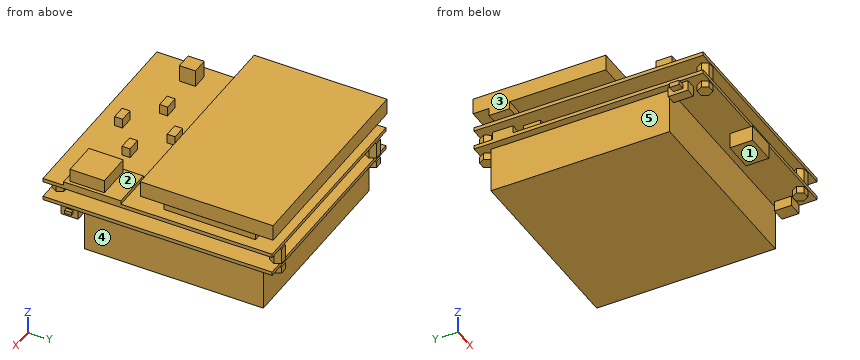
from build123d import *

# Parameters (mm, degrees)
SKETCH001_W   = 91
SKETCH001_H   = 100
PAD_DEPTH     = 1.6
SKETCH002_W   = 84.4
SKETCH002_H   = 78
PAD001_DEPTH  = 20
SKETCH003_W   = 13
SKETCH003_H   = 10
PAD002_DEPTH  = 6.8
SKETCH004_W   = 4.3
SKETCH004_H   = 8.6
PAD003_DEPTH  = 4.6
SKETCH005_W   = 6
SKETCH005_H   = 7.4
PAD004_DEPTH  = 4.4
SKETCH006_W   = 4.2
SKETCH006_H   = 2
PAD005_DEPTH  = 3
SKETCH007_W   = 3
SKETCH007_H   = 1.5
PAD006_DEPTH  = 1.4
PAD007_DEPTH  = 7
SKETCH009_W   = 7
SKETCH009_H   = 9
PAD008_DEPTH  = 3.4
SKETCH010_W   = 5
SKETCH010_H   = 7.4
PAD009_DEPTH  = 2.6
SKETCH011_W   = 91
SKETCH011_H   = 100
PAD010_DEPTH  = 1.6
SKETCH012_W   = 40
SKETCH012_H   = 4
SKETCH012_W_2 = 4
SKETCH012_H_2 = 40
PAD011_DEPTH  = 7.8
SKETCH013_W   = 91
SKETCH013_H   = 58
PAD012_DEPTH  = 7
SKETCH014_W   = 7
SKETCH014_H   = 9
PAD013_DEPTH  = 3.4
PAD014_DEPTH  = 3
SKETCH035_W   = 6
SKETCH035_H   = 3.5
PAD021_DEPTH  = 4.2
SKETCH036_W   = 7
SKETCH036_H   = 7
PAD022_DEPTH  = 7.4
SKETCH037_W   = 18
SKETCH037_H   = 25
PAD023_DEPTH  = 1.6
SKETCH038_W   = 15
SKETCH038_H   = 15
PAD024_DEPTH  = 5.8


with BuildPart() as part:
    # Sketch001 → Pad (new body)
    with BuildSketch(Plane.XY):
        Rectangle(SKETCH001_W, SKETCH001_H)
    extrude(amount=PAD_DEPTH)

    # Sketch002 (on Face5 of Pad) → Pad001 (join)
    with BuildSketch(Plane(origin=(0, 0, 0), x_dir=(1, 0, 0), z_dir=(0, 0, -1))):
        with Locations((0, -5.4)):
            Rectangle(SKETCH002_W, SKETCH002_H)
    extrude(amount=PAD001_DEPTH)

    # Sketch003 (on Face4 of Pad001) → Pad002 (join)
    with BuildSketch(Plane(origin=(0, 0, 0), x_dir=(1, 0, 0), z_dir=(0, 0, -1))):
        with Locations((-0.5, 45.6)):
            Rectangle(SKETCH003_W, SKETCH003_H)
    extrude(amount=PAD002_DEPTH)

    # Sketch004 (on Face4 of Pad002) → Pad003 (join)
    with BuildSketch(Plane(origin=(0, 0, 0), x_dir=(1, 0, 0), z_dir=(0, 0, -1))):
        with Locations((-41.95, 38.3)):
            Rectangle(SKETCH004_W, SKETCH004_H)
    extrude(amount=PAD003_DEPTH)

    # Sketch005 (on Face4 of Pad003) → Pad004 (join)
    with BuildSketch(Plane(origin=(0, 0, 0), x_dir=(1, 0, 0), z_dir=(0, 0, -1))):
        with Locations((41.9, 38.7)):
            Rectangle(SKETCH005_W, SKETCH005_H)
    extrude(amount=PAD004_DEPTH)

    # Sketch006 (on Face14 of Pad004) → Pad005 (join)
    with BuildSketch(Plane(origin=(-44.1, 0, 0), x_dir=(0, -1, 0), z_dir=(-1, 0, 0))):
        with Locations((38.3, -2)):
            Rectangle(SKETCH006_W, SKETCH006_H)
    extrude(amount=PAD005_DEPTH)

    # Sketch007 (on Face12 of Pad005) → Pad006 (join)
    with BuildSketch(Plane.YZ.offset(44.9)):
        with Locations((-38.7, -1.75)):
            Rectangle(SKETCH007_W, SKETCH007_H)
    extrude(amount=PAD006_DEPTH)

    # Sketch008 (on Face5 of Pad006) → Pad007 (join)
    with BuildSketch(Plane.XY.offset(1.6)):
        Polygon((-40, 45.401924), (-37, 45.401924), (-35.5, 48), (-37, 50.598076), (-40, 50.598076), (-41.5, 48), align=None)
        Polygon((39, 45.401924), (40.5, 48), (39, 50.598076), (36, 50.598076), (34.5, 48), (36, 45.401924), align=None)
        Polygon((-37, -49.598076), (-35.5, -47), (-37, -44.401924), (-40, -44.401924), (-41.5, -47), (-40, -49.598076), align=None)
        Polygon((39, -49.598076), (40.5, -47), (39, -44.401924), (36, -44.401924), (34.5, -47), (36, -49.598076), align=None)
    extrude(amount=PAD007_DEPTH)

    # Sketch009 (on Face5 of Pad007) → Pad008 (join)
    with BuildSketch(Plane.XY.offset(1.6)):
        with Locations((-42, 37.5)):
            Rectangle(SKETCH009_W, SKETCH009_H)
    extrude(amount=PAD008_DEPTH)

    # Sketch010 (on Face5 of Pad008) → Pad009 (join)
    with BuildSketch(Plane.XY.offset(1.6)):
        with Locations((-42, 25.3)):
            Rectangle(SKETCH010_W, SKETCH010_H)
    extrude(amount=PAD009_DEPTH)

    # Sketch011 (on Face74 of Pad009) → Pad010 (join)
    with BuildSketch(Plane.XY.offset(8.6)):
        Rectangle(SKETCH011_W, SKETCH011_H)
    extrude(amount=PAD010_DEPTH)

    # Sketch012 (on Face81 of Pad010) → Pad011 (join)
    with BuildSketch(Plane.XY.offset(10.2)):
        with Locations((0, 44)):
            Rectangle(SKETCH012_W, SKETCH012_H)
        with Locations((38.5, 20)):
            Rectangle(SKETCH012_W_2, SKETCH012_H_2)
    extrude(amount=PAD011_DEPTH)

    # Sketch013 (on Face91 of Pad011) → Pad012 (join)
    with BuildSketch(Plane.XY.offset(18)):
        with Locations((1, 22)):
            Rectangle(SKETCH013_W, SKETCH013_H)
    extrude(amount=PAD012_DEPTH)

    # Sketch014 (on Face4 of Pad012) → Pad013 (join)
    with BuildSketch(Plane(origin=(0, 0, 18), x_dir=(1, 0, 0), z_dir=(0, 0, -1))):
        with Locations((-41, -39.5)):
            Rectangle(SKETCH014_W, SKETCH014_H)
    extrude(amount=PAD013_DEPTH)

    # Sketch015 (on Face66 of Pad013) → Pad014 (join)
    with BuildSketch(Plane(origin=(0, 0, 0), x_dir=(1, 0, 0), z_dir=(0, 0, -1))):
        Polygon((-35.5, 47), (-37, 49.598076), (-40, 49.598076), (-41.5, 47), (-40, 44.401924), (-37, 44.401924), align=None)
        Polygon((39, 44.401924), (40.5, 47), (39, 49.598076), (36, 49.598076), (34.5, 47), (36, 44.401924), align=None)
        Polygon((-37, -50.598076), (-35.5, -48), (-37, -45.401924), (-40, -45.401924), (-41.5, -48), (-40, -50.598076), align=None)
        Polygon((39, -50.598076), (40.5, -48), (39, -45.401924), (36, -45.401924), (34.5, -48), (36, -50.598076), align=None)
    extrude(amount=PAD014_DEPTH)

    # Sketch035 (on Face20 of Pad014) → Pad021 (join)
    with BuildSketch(Plane.XY.offset(10.2)):
        with Locations((-15, -28.75)):
            Rectangle(SKETCH035_W, SKETCH035_H)
        with Locations((0, -17.25)):
            Rectangle(SKETCH035_W, SKETCH035_H)
        with Locations((15, -28.75)):
            Rectangle(SKETCH035_W, SKETCH035_H)
        with Locations((0, -40.25)):
            Rectangle(SKETCH035_W, SKETCH035_H)
    extrude(amount=PAD021_DEPTH)

    # Sketch036 (on Face20 of Pad021) → Pad022 (join)
    with BuildSketch(Plane.XY.offset(10.2)):
        with Locations((-37, -30.1)):
            Rectangle(SKETCH036_W, SKETCH036_H)
    extrude(amount=PAD022_DEPTH)

    # Sketch037 (on Face20 of Pad022) → Pad023 (join)
    with BuildSketch(Plane.XY.offset(10.2)):
        with Locations((36.5, -28.5)):
            Rectangle(SKETCH037_W, SKETCH037_H)
    extrude(amount=PAD023_DEPTH)

    # Sketch038 (on Face50 of Pad023) → Pad024 (join)
    with BuildSketch(Plane.XY.offset(11.8)):
        with Locations((36.5, -31.5)):
            Rectangle(SKETCH038_W, SKETCH038_H)
    extrude(amount=PAD024_DEPTH)


solid = part.part
Can you work these out from the model? Positions are in its coordinate system, mm. Face numbers are marked on the shaded views. A direction names the side the tool comes from. Round coordinates to 2 decimals unless told otherwise and drop trailing zeros. Order: outer loops, then holes, each group sorted by start corner. A loop starts at its lowest first (then second) coordinate and runs counter-clockwise, first axis right, second up. Notation, with made-up numbers: (18, 60.25) - (23, 60.25) arc R17 ccw to (23, 70.25) - close; hole circle Ø9 at (15.25, 19). An arc over 180 degrees is marked (long way). Answer in a Markdown table with one row per item.
(1) Suppose I cut it at B-B, the plane x = 22. Please give me the cut outline in (y, z).
From the geometry:
| item | result |
|---|---|
| outline | (-50, 0) - (-33.6, 0) - (-33.6, -20) - (44.4, -20) - (44.4, 0) - (50, 0) - (50, 1.6) - (-50, 1.6) - close; (-50, 8.6) - (50, 8.6) - (50, 10.2) - (-50, 10.2) - close; (-7, 18) - (51, 18) - (51, 25) - (-7, 25) - close |
(2) Suppose I cut it at C-C, the plane y = 8. Please give me the cut outline in (x, z).
From the geometry:
| item | result |
|---|---|
| outline | (-45.5, 0) - (-42.2, 0) - (-42.2, -20) - (42.2, -20) - (42.2, 0) - (45.5, 0) - (45.5, 1.6) - (-45.5, 1.6) - close; (-45.5, 8.6) - (45.5, 8.6) - (45.5, 10.2) - (40.5, 10.2) - (40.5, 18) - (46.5, 18) - (46.5, 25) - (-44.5, 25) - (-44.5, 18) - (36.5, 18) - (36.5, 10.2) - (-45.5, 10.2) - close |
(3) For P1, Ø3, axis at y = 25.5, z = 3, coming from the +X side; P2, Ø4, axis at y = 37.5, z = 11, coming from the -X side; P3, Ø0.8, axis at x = 4.5, z = 1, coming from the +Y side, each with a flat end and sliding along its axis, tell me the tip position at first contact or that it passes through.
From the geometry:
| item | result |
|---|---|
| P1 | stops at x = 45.5 |
| P2 | stops at x = -45.5 |
| P3 | stops at y = 50 |
(4) Suppose I cut it at A-A, the plane y = 38.5. Please give me the cut outline in (x, z).
From the geometry:
| item | result |
|---|---|
| outline | (-45.5, 0) - (-42.2, 0) - (-42.2, -20) - (42.2, -20) - (42.2, 0) - (45.5, 0) - (45.5, 1.6) - (-38.5, 1.6) - (-38.5, 5) - (-45.5, 5) - close; (-45.5, 8.6) - (45.5, 8.6) - (45.5, 10.2) - (40.5, 10.2) - (40.5, 18) - (46.5, 18) - (46.5, 25) - (-44.5, 25) - (-44.5, 14.6) - (-37.5, 14.6) - (-37.5, 18) - (36.5, 18) - (36.5, 10.2) - (-45.5, 10.2) - close |
(5) If we mould it in two halves opening along Y, with no side actions, what happens to the marked faces 1 and 2? For each: released by +Y, released by -Y, zero draft, split by the parting line, or undercut.
From the geometry:
| item | result |
|---|---|
| face 1 | zero draft |
| face 2 | undercut |
(6) Suppose I cut it at D-D, the plane z = -15. Please give me the cut outline in (x, y).
From the geometry:
| item | result |
|---|---|
| outline | (-42.2, -33.6) - (42.2, -33.6) - (42.2, 44.4) - (-42.2, 44.4) - close |
(7) Please list where these lines run through material, in increasing order: L1, parallel to Z at x = -26, y = 38; L2, parallel to Y at x = -2, z = 11; L3, parallel to Z at x = -32, y = 44.5. Write a range as from..to.
From the geometry:
| item | result |
|---|---|
| L1 | z = -20..1.6, 8.6..10.2, 18..25 |
| L2 | y = -42..-38.5, -19..-15.5, 42..46 |
| L3 | z = 0..1.6, 8.6..10.2, 18..25 |
(8) Which directions (+Z, -Z, +X, -X, +Y, -Y) give clear straight access to the entire face, cutting with the end or side of a thin tool? Please do the marked faces 3, 4 and 5.
From the geometry:
| item | result |
|---|---|
| face 3 | +Z, -X, +Y, -Y |
| face 4 | -Z, +X, +Y |
| face 5 | -Z, -X, +Y |
